Read the model definition and answer for the solid it produces. Units are mm, in the model's axes. Face numbers are marked on the shaded views. A direction names the side the tool comes from. Coordinates: 2 decimals unless noted, no trailing zeros. Write each loop counter-clockwise with the first axis right and the second up, starting at its lowest first coordinate (ties: lowest second). Pieces come first, ordered by that corner, then holes.
(1) Section A-A on y = -140.5 is taken. Write down the section's boundary in (x, z).
(2) Section D-D on y = 174.5 is taken. Write down the section's boundary in (x, z).
(3) The mould has two halves that part along X. Classify the marked faces 4, 5 and 6: +X half, -X half, draft (parallel to the pull), parting line (faces both ways), or undercut.
(4) Which of the six approach directions +Z, -Z, +X, -X, +Y, -Y give full straight-line access (tool end or side, diameter ignored) to the marked faces 1, 2 and 3?
(5) Section B-B on z = 51.5 is taken. Write down the section's boundary in (x, y).
(6) Given pin 1 (2 mm diameter, centred on y = -83.5, z = -39, fed in from +X); pin 2 (4.5 mm diameter, centred on x = 42.5, y = 205.5, fed in from -Z); pin 3 (22 mm diameter, centred on x = 163, y = 220, fed in from +Z), each flat-ended and moving along its own axis, determine where each tip first touches the part or whether it passes through.
(7) Section C-C on x = 158.5 is taken. Write down the section's boundary in (y, z).
(8) Find the intervals of material crossed by probe 1 along X at (y, z) = (-144, -26); probe 2 along Z at (x, y) = (146, 10), in increasing order.
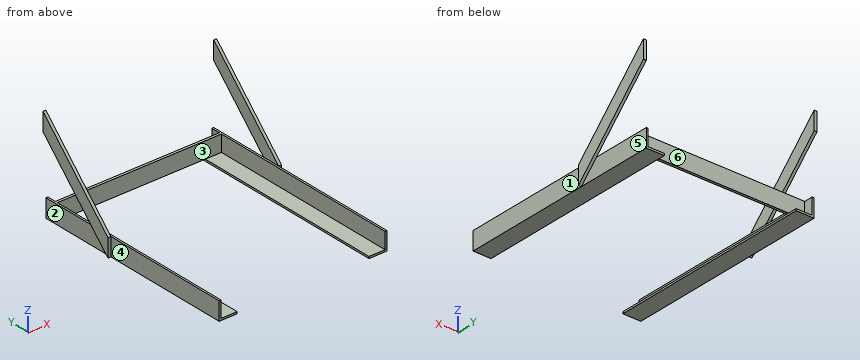
from build123d import *

# Parameters (mm, degrees)
F0_W     = 4.191
F0_H     = 35.941
F0_W_2   = 35.687
F0_H_2   = 4.191
F1_DEPTH = 228.6
F2_W     = 35.687
F2_H     = 5.588
F2_W_2   = 291.719
F3_DEPTH = 35.941
F5_DEPTH = 6.35


with BuildPart() as f1:
    # F0 (on Front) → F1 (new body, symmetric)
    with BuildSketch(Plane.XZ):
        with Locations((-183.642, -17.9705)):
            Rectangle(F0_W, F0_H)
        with Locations((-163.703, -38.0365)):
            Rectangle(F0_W_2, F0_H_2)
        with Locations((-183.642, -38.0365)):
            Rectangle(F0_W, F0_H_2)
    extrude(amount=F1_DEPTH, both=True)



with BuildPart() as f1b:
    # F0 (on Front) → F1, piece 2 (new body, symmetric)
    with BuildSketch(Plane.XZ):
        with Locations((183.642, -17.9705)):
            Rectangle(F0_W, F0_H)
        with Locations((183.642, -38.0365)):
            Rectangle(F0_W, F0_H_2)
        with Locations((163.703, -38.0365)):
            Rectangle(F0_W_2, F0_H_2)
    extrude(amount=F1_DEPTH, both=True)


with BuildPart() as f1_1:
    add(f1.part)

    add(f1b.part)  # F3 merges F1b
    # F2 (on face) → F3 (join)
    with BuildSketch(Plane.XY.offset(-35.941)):
        with Locations((-163.703, 205.994)):
            Rectangle(F2_W, F2_H)
        with Locations((0, 205.994)):
            Rectangle(F2_W_2, F2_H)
        with Locations((163.703, 205.994)):
            Rectangle(F2_W, F2_H)
    extrude(amount=F3_DEPTH)

    # F4 (on face) → F5 (join)
    with BuildSketch(Plane.YZ.offset(185.7375)):
        Polygon((228.6, 171.45), (57.15, 0), (97.282, 0), (228.6, 131.318), align=None)
        Polygon((97.282, 0), (57.15, 0), (57.15, -40.132), align=None)
    extrude(amount=F5_DEPTH)

    # F6: F1 across plane


with BuildPart() as f1_2:
    add(f1_1.part)
    add(f1_1.part.mirror(Plane.YZ))


solid = f1_2.part
Response:
1. outline: (-185.74, -40.13) - (-145.86, -40.13) - (-145.86, -35.94) - (-181.55, -35.94) - (-181.55, 0) - (-185.74, 0) - close; (145.86, -40.13) - (185.74, -40.13) - (185.74, 0) - (181.55, 0) - (181.55, -35.94) - (145.86, -35.94) - close
2. outline: (-192.09, 77.22) - (-185.74, 77.22) - (-185.74, 117.35) - (-192.09, 117.35) - close; (-185.74, -40.13) - (-145.86, -40.13) - (-145.86, -35.94) - (-181.55, -35.94) - (-181.55, 0) - (-185.74, 0) - close; (145.86, -40.13) - (185.74, -40.13) - (185.74, 0) - (181.55, 0) - (181.55, -35.94) - (145.86, -35.94) - close; (185.74, 77.22) - (192.09, 77.22) - (192.09, 117.35) - (185.74, 117.35) - close
3. face 4: -X half
3. face 5: +X half
3. face 6: undercut
4. face 1: +Z, -Z, +X, -Y
4. face 2: -Z, -X, +Y
4. face 3: +Z, -Y
5. outline: (-192.09, 108.65) - (-185.74, 108.65) - (-185.74, 148.78) - (-192.09, 148.78) - close; (185.74, 108.65) - (192.09, 108.65) - (192.09, 148.78) - (185.74, 148.78) - close
6. pin 1: stops at x = 185.74
6. pin 2: stops at z = -35.94
6. pin 3: stops at z = -35.94
7. outline: (-228.6, -40.13) - (228.6, -40.13) - (228.6, -35.94) - (208.79, -35.94) - (208.79, 0) - (203.2, 0) - (203.2, -35.94) - (-228.6, -35.94) - close
8. probe 1: x = -185.74 to -181.55, 181.55 to 185.74
8. probe 2: z = -40.13 to -35.94
